Geometry check sheet. Reference: the model listing, model coordinates, mm. A direction names the side the tool comes from. Coordinates: 2 decimals unless noted, no trailing zeros. Write each loop counter-clockwise with the first axis right and the second up, starting at its lowest first coordinate (ties: lowest second). Pieces come first, ordered by that corner, then holes. Notation, with made-up numbers: (4.25, 88) -> (61.25, 88) arc R26 cw to (61.25, 116) -> close; hole circle Ø11 at (38, 50.5). An arc over 180 degrees is marked (long way). One line per question, with ' | ' between items.
```python
from build123d import *

# Parameters (mm, degrees)
F0_W     = 20
F0_H     = 20
F0_W_2   = 16
F0_H_2   = 16
F1_DEPTH = 800
F2_R     = 5
F3_DEPTH = 20.001


with BuildPart() as f1:
    # F0 (on Front) → F1 (new body)
    with BuildSketch(Plane.XZ):
        with Locations((10, 10)):
            Rectangle(F0_W, F0_H)
        with Locations((10, 10)):
            Rectangle(F0_W_2, F0_H_2, mode=Mode.SUBTRACT)
    extrude(amount=F1_DEPTH)

    # F2 (on face) → F3 (cut, through all)
    with BuildSketch(Plane.YZ.offset(20)):
        with Locations((-790, 10)):
            Circle(F2_R)
        with Locations((-400, 10)):
            Circle(F2_R)
        with Locations((-10, 10)):
            Circle(F2_R)
    extrude(amount=-F3_DEPTH, mode=Mode.SUBTRACT)


solid = f1.part
```
(1) Draft check along X on faces 3 (the face through (20, -394, 10)), 4 (the face through (2, -394, 10)), 5 (the face through (1, -800, 10)). Enter one of: pulls with the +X half, pulls with the -X half, needs draft (parallel to the pull), parting line crosses it, or undercut.
Answers below:
face 3: pulls with the +X half | face 4: undercut | face 5: needs draft
(2) Material ranges on line 1 (Y direction, x = 19, z = 9.75); line 2 (Y direction, x = 18.75, z = 10.75); line 3 (X direction, y = -636, z = 10.75), recorded low to high.
Answers below:
line 1: y = -800 to -794.99, -785.01 to -404.99, -395.01 to -14.99, -5.01 to 0 | line 2: y = -800 to -794.94, -785.06 to -404.94, -395.06 to -14.94, -5.06 to 0 | line 3: x = 0 to 2, 18 to 20
(3) Tool access check on faces 1 (the face through (10, -394, 18)), 2 (the face through (10, -394, 0)). Record the directions out of +Z, -Z, +X, -X, +Y, -Y that give a thin tool (end or side, any length) a straight path to the whole face; none if there is none.
Answers below:
face 1: +Y, -Y | face 2: -Z, +X, -X, +Y, -Y
(4) Cross-section at B-B (x = 8). Record the cut outline in (y, z), plus the area to 3 significant figures.
Answers below:
outline: (-800, 0) -> (0, 0) -> (0, 2) -> (-800, 2) -> close; (-800, 18) -> (0, 18) -> (0, 20) -> (-800, 20) -> close | area: 3,200 mm²
(5) Cross-section at C-C (y = -691). Record the cut outline in (x, z).
Answers below:
outline: (0, 0) -> (20, 0) -> (20, 20) -> (0, 20) -> close; hole (2, 2) -> (18, 2) -> (18, 18) -> (2, 18) -> close
(6) Cross-section at A-A (z = 10). Count the separate pieces of the cut face and the enclosed holes in it, plus the area to 3 significant figures.
Answers below:
separate pieces: 8 | enclosed holes: 0 | area: 3,080 mm²
